Can you work these out from the model? Positions are in its coordinate system, mm. A direction names the side the tool comes from. Round coordinates to 2 decimals unless told otherwise and drop trailing zeros. Loops run counter-clockwise (first coordinate to the right, second up) from the corner with the lowest first, then second, coordinate; pieces in that order, holes last. Notation, with made-up numbers: (40.5, -10) -> (52.5, -10) arc R23 ccw to (52.5, -2) -> close; hole circle Ø11 at (83, 16.25). An arc over 180 degrees is marked (long way). Use a Markdown table: item, result.
from build123d import *

# Parameters (mm, degrees)
BOSS_EXTRUDE1_DEPTH = 25.4
FILLET1_R           = 2.54
FILLET2_R           = 5.715
SKETCH2_W           = 191.77
SKETCH2_H           = 5.715
CUT_EXTRUDE1_DEPTH  = 12.7
CUT_EXTRUDE2_REACH  = 260.91
SKETCH3_W           = 25.4
SKETCH3_H           = 6.35


with BuildPart() as part:
    # Sketch1 → Boss-Extrude1 (new body)
    with BuildSketch(Plane(origin=(0, 0, 0), x_dir=(1, 0, 0), z_dir=(0, 1, 0))):
        Polygon((-92.71, 0), (92.71, 0), (92.71, -168.91), (41.91, -168.91), (41.91, -172.085), (95.885, -172.085), (95.885, 3.175), (-95.885, 3.175), (-95.885, -172.085), (-41.91, -172.085), (-41.91, -168.91), (-92.71, -168.91), align=None)
    extrude(amount=BOSS_EXTRUDE1_DEPTH)

    # Fillet1
    fillet1_edges = [part.edges().sort_by_distance(p)[0] for p in [
        (92.71, 12.7, 168.91),
        (92.71, 12.7, 0),
        (-92.71, 12.7, 0),
        (-92.71, 12.7, 168.91),
    ]]
    fillet(fillet1_edges, radius=FILLET1_R)

    # Fillet2
    fillet2_edges = [part.edges().sort_by_distance(p)[0] for p in [
        (-95.885, 12.7, -3.175),
        (95.885, 12.7, -3.175),
        (95.885, 12.7, 172.085),
        (-95.885, 12.7, 172.085),
    ]]
    fillet(fillet2_edges, radius=FILLET2_R)

    # Sketch2 → Cut-Extrude1 (cut)
    with BuildSketch(Plane(origin=(0, 25.4, 0), x_dir=(1, 0, 0), z_dir=(0, 1, 0))):
        with Locations((0, -169.2275)):
            Rectangle(SKETCH2_W, SKETCH2_H)
    extrude(amount=-CUT_EXTRUDE1_DEPTH, mode=Mode.SUBTRACT)

    # Cut-Extrude2: up to this face of the body (flat: up to its plane)
    cut_extrude2_end = Plane(part.part.faces().sort_by_distance((95.885, 12.7, 84.455))[0])
    # Sketch3 → Cut-Extrude2 (cut, up to the picked face)
    with BuildSketch(Plane.ZY.offset(95.885), mode=Mode.PRIVATE) as cut_extrude2_sk1:
        with Locations((140.97, 12.7)):
            Rectangle(SKETCH3_W, SKETCH3_H)
    cut_extrude2_tool1 = split(extrude(cut_extrude2_sk1.sketch, amount=-CUT_EXTRUDE2_REACH, mode=Mode.PRIVATE), bisect_by=cut_extrude2_end, keep=Keep.BOTH, mode=Mode.PRIVATE)
    add(cut_extrude2_tool1.solids().sort_by(Axis((-95.885, 12.7, 140.97), (1, 0, 0)))[0], mode=Mode.SUBTRACT)


solid = part.part
1. I want a section at A-A (x = -51). Please give me the cut outline in (y, z) (3 decimals).
Answer sheet:
| item | result |
|---|---|
| outline | (0, -3.175) -> (25.4, -3.175) -> (25.4, 0) -> (0, 0) -> close; (0, 168.91) -> (12.7, 168.91) -> (12.7, 172.085) -> (0, 172.085) -> close |
2. If we mould it in two halves opening along Y, with no side actions, what happens to faces 1 (the flat face through (-43.1, 0, -0.3)), 2 (the flat face through (69, 12.7, 170)), 3 (the cylindrical face through (94.255, 12.878, -1.456))? For each: +Y half, -Y half, draft (parallel to the pull), parting line (faces both ways), or undercut.
Answer sheet:
| item | result |
|---|---|
| face 1 | -Y half |
| face 2 | +Y half |
| face 3 | draft |
3. I want a section at C-C (y = 6). Please give me the cut outline in (x, z) (3 decimals).
Answer sheet:
| item | result |
|---|---|
| outline | (-95.885, 2.54) arc R5.715 ccw to (-90.17, -3.175) -> (90.17, -3.175) arc R5.715 ccw to (95.885, 2.54) -> (95.885, 166.37) arc R5.715 ccw to (90.17, 172.085) -> (41.91, 172.085) -> (41.91, 168.91) -> (90.17, 168.91) arc R2.54 cw to (92.71, 166.37) -> (92.71, 2.54) arc R2.54 cw to (90.17, 0) -> (-90.17, 0) arc R2.54 cw to (-92.71, 2.54) -> (-92.71, 166.37) arc R2.54 cw to (-90.17, 168.91) -> (-41.91, 168.91) -> (-41.91, 172.085) -> (-90.17, 172.085) arc R5.715 ccw to (-95.885, 166.37) -> close |
4. I want a section at D-D (y = 22). Please give me the cut outline in (x, z) (3 decimals), plus the area to 3 significant figures.
Answer sheet:
| item | result |
|---|---|
| outline | (-95.885, 2.54) arc R5.715 ccw to (-90.17, -3.175) -> (90.17, -3.175) arc R5.715 ccw to (95.885, 2.54) -> (95.885, 166.37) -> (92.71, 166.37) -> (92.71, 2.54) arc R2.54 cw to (90.17, 0) -> (-90.17, 0) arc R2.54 cw to (-92.71, 2.54) -> (-92.71, 166.37) -> (-95.885, 166.37) -> close |
| area | 1,650 mm² |
5. Will these pins go through, and if not, where does the flat tip stop? pin 1 Ø1 at (x, y) = (95, 21) entering from +Z; pin 2 Ø6.5 at (x, z) = (75.5, 168) entering from +Y; pin 3 Ø3.5 at (x, y) = (94, 11.5) entering from +Z.
Answer sheet:
| item | result |
|---|---|
| pin 1 | stops at z = 166.37 |
| pin 2 | stops at y = 12.7 |
| pin 3 | stops at z = 171.69 |
6. Which directions (+Z, -Z, +X, -X, +Y, -Y) give clear straight access to the entire face, cutting with the end or side of a thin tool? Please do faces 4 (the flat face through (-1, 13, 0)), 5 (the flat face through (-69, 12.7, 170)), 6 (the flat face through (95.885, 13, 86)).
Answer sheet:
| item | result |
|---|---|
| face 4 | +Y, -Y |
| face 5 | +Z, +X, -X, +Y |
| face 6 | +Z, -Z, +X, +Y, -Y |
7. I want a section at B-B (z = 120.5). Please give me the cut outline in (x, y) (3 decimals), plus the area to 3 significant figures.
Answer sheet:
| item | result |
|---|---|
| outline | (-95.885, 0) -> (-92.71, 0) -> (-92.71, 25.4) -> (-95.885, 25.4) -> close; (92.71, 0) -> (95.885, 0) -> (95.885, 25.4) -> (92.71, 25.4) -> close |
| area | 161 mm² |
8. I need wall thicknesses on line 1 (X direction, y = 18, z = 112) (3 decimals); line 2 (Z direction, x = -80.5, y = 5.5) (3 decimals); line 3 (Z direction, x = 81, y = 14.5) (3 decimals). Which ranges of each line are inside material? Lowest first, please.
Answer sheet:
| item | result |
|---|---|
| line 1 | x = -95.885 to -92.71, 92.71 to 95.885 |
| line 2 | z = -3.175 to 0, 168.91 to 172.085 |
| line 3 | z = -3.175 to 0 |
